Autodesk Inventor part; units mm, degrees
ref_plane "YZ Plane" through (0, 0, 0) normal (1, 0, 0) x (0, 1, 0)
ref_plane "XZ Plane" through (0, 0, 0) normal (0, 1, 0) x (-1, 0, 0)
ref_plane "XY Plane" through (0, 0, 0) normal (0, 0, 1) x (1, 0, 0)
sketch "スケッチ1" plane through (0, 0, 0) normal (0, 1, 0) x (-1, 0, 0)
  line L0 (55, 0) -> (0, 0)
  line L1 (0, 0) -> (0, -20)
  line L2 (0, -20) -> (55, -20)
  line L3 (55, -20) -> (55, 0)
  dimension "d0" = 20
  dimension "d1" = 55
extrude "押し出し1" add sketch "スケッチ1" along normal blind 1.5
sketch "スケッチ2" plane through (0, 0, 0) normal (0, -1, 0) x (1, 0, 0)
  line L0 (-7, -10.1005) -> (0, -20)
  line L1 (-7, -10.1005) -> (-48, -10.1005)
  line L2 (0, -20) -> (-55, -20)
  line L3 (-48, -10.1005) -> (-55, -20)
  line L4 (0, 0) -> (0, -20)
  line L5 (-55, 0) -> (0, 0)
  line L6 (-55, -20) -> (-55, 0)
  line L7 (0, -20) -> (-55, -20)
  point P0 (0, -20)
extrude "押し出し2" cut sketch "スケッチ2" against normal through all contours L1 L3 L6 L5 L4 L0
fillet "フィレット1" radius 1 4 edges at (-7, 0.75, -10.1005) (0, 0.75, -20) (-48, 0.75, -10.1005) (-55, 0.75, -20)
sketch "スケッチ3" plane through (0, 0, 0) normal (0, -1, 0) x (1, 0, 0)
  arc A0 (-53.8846, -18.4226) -> (-53.0681, -20) centre (-53.0681, -19) ccw
  line L0 (-1.9319, -20) -> (-53.0681, -20)
  arc A1 (-1.9319, -20) -> (-1.1154, -18.4226) centre (-1.9319, -19) ccw
  line L1 (-1.1154, -18.4226) -> (-6.7011, -10.5232)
  arc A2 (-6.7011, -10.5232) -> (-7.5176, -10.1005) centre (-7.5176, -11.1005) ccw
  line L2 (-7.5176, -10.1005) -> (-47.4824, -10.1005)
  arc A3 (-47.4824, -10.1005) -> (-48.2989, -10.5232) centre (-47.4824, -11.1005) ccw
  line L3 (-48.2989, -10.5232) -> (-53.8846, -18.4226)
  circle A4 centre (-46.9647, -12.1005) radius 0.8
  circle A5 centre (-8.0353, -12.1005) radius 0.8
  circle A6 centre (-3.8637, -18) radius 0.8
  circle A7 centre (-51.1363, -18) radius 0.8
  circle A8 centre (-27.5, 18.8909) radius 46.7105
  line L4 (-27.5, 18.8909) -> (-54.4683, -19.2481)
  line L5 (-27.5, 18.8909) -> (-0.5317, -19.2481)
  arc A9 (-53.8846, -18.4226) -> (-53.0681, -20) centre (-53.0681, -19) ccw
  line L6 (-27.5, 18.8909) -> (-49.0163, -22.569)
  line L7 (-27.5, 18.8909) -> (-43.1624, -25.1155)
  line L8 (-27.5, 18.8909) -> (-37.016, -26.84)
  line L9 (-27.5, 18.8909) -> (-30.6919, -27.7104)
  line L10 (-27.5, 18.8909) -> (-24.3081, -27.7104)
  line L11 (-27.5, 18.8909) -> (-17.984, -26.84)
  line L12 (-27.5, 18.8909) -> (-11.8376, -25.1155)
  line L13 (-27.5, 18.8909) -> (-5.9837, -22.569)
  line L14 (-46.9647, -12.1005) -> (-8.0353, -12.1005)
  line L15 (-51.1363, -18) -> (-3.8637, -18)
  line L16 (-46.9647, -12.1005) -> (-51.1363, -18)
  line L17 (-8.0353, -12.1005) -> (-3.8637, -18)
  circle A10 centre (-46.9647, -12.1005) radius 3.0011
  circle A11 centre (-51.1363, -18) radius 3.9863
  circle A12 centre (-8.0353, -12.1005) radius 3.0011
  circle A13 centre (-3.8637, -18) radius 3.9863
  line L18 (-43.5835, -12.1005) -> (-38.5302, -12.1005)
  point P0 (0, 0)
  point P1 (-14.37, -18)
  point P2 (-8.3548, -18)
  point P3 (-11.4165, -12.1005)
  point P4 (-16.4698, -12.1005)
  point P5 (-24.9732, -18)
  point P6 (-19.8235, -18)
  point P7 (-21.0511, -12.1005)
  point P8 (-25.3773, -12.1005)
  point P9 (-35.1765, -18)
  point P10 (-30.0268, -18)
  point P11 (-29.6227, -12.1005)
  point P12 (-33.9489, -12.1005)
  point P13 (-46.6452, -18)
  point P14 (-40.63, -18)
  dimension "d7" = 1.6
  dimension "d8" = 1.6
  dimension "d9" = 1.6
  dimension "d10" = 1.6
  dimension "d11" = 2
  dimension "d12" = 2
  dimension "d13" = 2
  dimension "d14" = 2
  dimension "d15" = 2
  dimension "d16" = 2
  dimension "d19" = 7.837
  dimension "d20" = 7.837
  dimension "d21" = 7.837
  dimension "d22" = 7.837
  dimension "d25" = 7.837
  dimension "d26" = 7.837
  dimension "d27" = 7.837
  dimension "d28" = 7.837
  dimension "d29" = 7.837
extrude "押し出し3" cut sketch "スケッチ3" against normal through all contours L16 L15 A7 | A7 L15 L16 | L16 L14 A4 | A4 L14 L16 | L6 L14 L7 L15 | L8 L14 L9 L15 | L14 L11 L15 L10 | L14 L13 L15 L12 | L14 L17 A5 | A5 L17 L14 | L17 L15 A6 | A6 L15 L17
fillet "フィレット2" radius 2 16 edges at (-43.5835, 0.75, -12.1005) (-38.5302, 0.75, -12.1005) (-46.6452, 0.75, -18) (-40.63, 0.75, -18) (-33.9489, 0.75, -12.1005) (-29.6227, 0.75, -12.1005) (-35.1765, 0.75, -18) (-30.0268, 0.75, -18) (-24.9732, 0.75, -18) (-25.3773, 0.75, -12.1005) (-21.0511, 0.75, -12.1005) (-19.8235, 0.75, -18) (-11.4165, 0.75, -12.1005) (-8.3548, 0.75, -18) (-14.37, 0.75, -18) (-16.4698, 0.75, -12.1005)
equation "\"d12\" = d11"
equation "\"d13\" = d11"
equation "\"d14\" = d11"
equation "\"d15\" = d11"
equation "\"d16\" = d11"
equation "\"d19\" = d29"
equation "\"d20\" = d19"
equation "\"d21\" = d19"
equation "\"d22\" = d19"
equation "\"d25\" = d19"
equation "\"d26\" = d19"
equation "\"d27\" = d19"
equation "\"d28\" = d19"
properties part number "shield_side_side" material "アルミニウム 6061"
Part model, mm, in its own coordinate system. A direction names the side the tool comes from. Coordinates: 2 decimals unless noted, no trailing zeros. Return JSON: item names as keys, results as strings.
1. 3-axis set-ups, long thin cutter, end or side, ignore diameter. For faces 1 (the face through (-25.167, 0.74, -15.174)), 2 (the face through (-27, 1.5, -15)): which of +Z, -Z, +X, -X, +Y, -Y reach the whole face in a straight line?
Determined:
{"face 1": "+Y, -Y", "face 2": "+Z, -Z, +X, -X, +Y"}
2. Flat gauge pins, fed straight in: pin 1 Ø1.4 at (x, z) = (-3.86, -18) entering from -Y; pin 2 Ø1.8 at (x, z) = (-46.96, -12.1) entering from -Y. Where does each tip first touch, or does it go through?
Determined:
{"pin 1": "through", "pin 2": "y = 0"}
3. Saw through at A-A, the plane y = 0.25. Count the separate pieces of the cut face and the enclosed holes in it, then the cut area to 3 significant figures.
Determined:
{"separate pieces": "1", "enclosed holes": "8", "area": "361 mm²"}
4. Pull direction Z, two halves, no side cores. Call faces 3 (the face through (-3.947, 0.74, -14.418)), 4 (the face through (-27, 1, -20)), 5 (the face through (-21.43, 0.76, -12.54)): pulls with the +Z half, pulls with the -Z half, needs draft (parallel to the pull), parting line crosses it, or undercut.
Determined:
{"face 3": "pulls with the +Z half", "face 4": "pulls with the -Z half", "face 5": "undercut"}
5. Probe L1, parallel to Z at x = -42.5, y = 0.9; L2, parallel to X at y = 1.1, z = -14; L3, parallel to X at y = 0.95, z = -15.5. List the from-to ranges inside material, lowest first.
Determined:
{"L1": "-20 to -18, -12.1 to -10.1", "L2": "-50.76 to -44.57, -39.37 to -34.34, -29.77 to -25.23, -20.66 to -15.63, -10.43 to -4.24", "L3": "-51.82 to -45.29, -39.74 to -34.66, -29.86 to -25.14, -20.34 to -15.26, -9.71 to -3.18"}
